```python
from build123d import *

# Parameters (mm, degrees)
BASPROSKE_W        = 10
BASPROSKE_H        = 14
TOOTHCUT_DEPTH     = 23.181073013
TEETHCUTS_COUNT    = 26
TEETHCUTS_ANGLE    = 346.153846154
BORSKE_R           = 0.4
BORE_DEPTH         = 50.0000508
SKETCH1_R          = 8.54
CUT_EXTRUDE1_DEPTH = 5.5
SKETCH2_R          = 3.75
CUT_EXTRUDE2_DEPTH = 21.500522978
SKETCH3_R          = 15.294835459
CUT_EXTRUDE3_DEPTH = 2


with BuildPart() as part:
    # BasProSke → Base-Revolve (revolve)
    with BuildSketch(Plane(origin=(0, 0, 0), x_dir=(1, 0, 0), z_dir=(0, 1, 0)), mode=Mode.PRIVATE) as base_revolve_sk:
        with Locations((5, 7)):
            Rectangle(BASPROSKE_W, BASPROSKE_H)
    revolve(base_revolve_sk.sketch.rotate(Axis((-10, 0, 0), (1, 0, 0)), 180), axis=Axis((-10, 0, 0), (1, 0, 0)))

    # TooCutSke → ToothCut (cut, through all)
    with BuildSketch(Plane(origin=(0, 0, 0), x_dir=(0, 0, -1), z_dir=(1, 0, 0))):
        with BuildLine():
            ThreePointArc((0.476965065, 11.739314517), (0, 11.749), (-0.476965065, 11.739314517))
            ThreePointArc((-0.476965065, 11.739314517), (-0.82065865, 12.901686978), (-1.424117301, 13.952911348))
            ThreePointArc((-1.424117301, 13.952911348), (0, 14.0254), (1.424117301, 13.952911348))
            ThreePointArc((1.424117301, 13.952911348), (0.82065865, 12.901686978), (0.476965065, 11.739314517))
        make_face()
    toothcut = extrude(amount=TOOTHCUT_DEPTH, mode=Mode.SUBTRACT)

    # TeethCuts: ToothCut ×26 about axis
    teethcuts_axis = Axis((-10, 0, 0), (1, 0, 0))
    for i in range(1, TEETHCUTS_COUNT):
        add(toothcut.rotate(teethcuts_axis, i * TEETHCUTS_ANGLE / (TEETHCUTS_COUNT - 1)), mode=Mode.SUBTRACT)

    # BorSke → Bore (cut, symmetric)
    with BuildSketch(Plane(origin=(0, 0, 0), x_dir=(0, 0, -1), z_dir=(1, 0, 0))):
        with Locations(Location((0, 0, 0), (0, 0, 180))):
            Circle(BORSKE_R)
    extrude(amount=BORE_DEPTH, both=True, mode=Mode.SUBTRACT)

    # Sketch1 → Cut-Extrude1 (cut)
    with BuildSketch(Plane(origin=(10, 0, 0), x_dir=(0, 0, -1), z_dir=(1, 0, 0))):
        Circle(SKETCH1_R)
    extrude(amount=-CUT_EXTRUDE1_DEPTH, mode=Mode.SUBTRACT)

    # Sketch2 → Cut-Extrude2 (cut, through all)
    with BuildSketch(Plane(origin=(4.5, 0, 0), x_dir=(0, 0, -1), z_dir=(1, 0, 0))):
        Circle(SKETCH2_R)
    extrude(amount=-CUT_EXTRUDE2_DEPTH, mode=Mode.SUBTRACT)

    # Sketch3 → Cut-Extrude3 (cut)
    with BuildSketch(Plane.ZY):
        Circle(SKETCH3_R)
    extrude(amount=-CUT_EXTRUDE3_DEPTH, mode=Mode.SUBTRACT)


solid = part.part
```
Here's how the part is built. I have some questions about the finished solid (model axes, mm). A direction names the side the tool comes from. Round coordinates to 2 decimals unless told otherwise and drop trailing zeros. Loops run counter-clockwise (first coordinate to the right, second up) from the corner with the lowest first, then second, coordinate; pieces in that order, holes last. Notation, with made-up numbers: (5.25, 21) -> (50.25, 21) arc R13 cw to (50.25, 41) -> close; hole circle Ø5 at (-34, 81.25). An arc over 180 degrees is marked (long way). Answer as CSV lines item,"result".
1. For pin 1 (4 mm diameter, centred on x = 3.5, y = -9.5, fed in from -Z); pin 2 (8.5 mm diameter, centred on y = 0.5, z = 2.5, fed in from +X); pin 3 (3 mm diameter, centred on x = 8.5, z = 6, fed in from -Y), each with a flat end and sliding along its axis, tell me the tip position at first contact or that it passes through.
Final values:
pin 1,"stops at z = -10.66"
pin 2,"stops at x = 4.5"
pin 3,"stops at y = -13.19"
2. If we section it at B-B on y = -8: Please give me the cut outline in (x, z), plus the area to 3 significant figures.
Final values:
outline,"(2, -10.15) -> (10, -10.15) -> (10, -2.99) -> (4.5, -2.99) -> (4.5, 2.99) -> (10, 2.99) -> (10, 10.15) -> (2, 10.15) -> close"
area,"130 mm^2"
3. Thinking about a two-plate mould opening in Y: for faces 5 (the face through (5.944, -12.873, -0.808)), 6 (the face through (5.944, 11.774, -5.266)), which applies, released by +Y, released by -Y, zero draft, split by the parting line, or undercut?
Final values:
face 5,"released by -Y"
face 6,"undercut"
4. If we section it at A-A on z = 0: Please give me the cut outline in (x, y), plus the area to 3 significant figures.
Final values:
outline,"(2, -11.75) -> (10, -11.75) -> (10, -8.54) -> (4.5, -8.54) -> (4.5, -3.75) -> (2, -3.75) -> close; (2, 3.75) -> (4.5, 3.75) -> (4.5, 8.54) -> (10, 8.54) -> (10, 11.75) -> (2, 11.75) -> close"
area,"75.3 mm^2"
5. If I drill on L1, parallel to Y at x = 6.85, z = 0; L2, parallel to Y at x = 2.7, z = 0; L3, parallel to Y at x = 8.25, z = -12, over which ranges is the centre line in solid material (lowest first)?
Final values:
L1,"y = -11.75 to -8.54, 8.54 to 11.75"
L2,"y = -11.75 to -3.75, 3.75 to 11.75"
L3,"y = -6.76 to -5.58, -3.81 to -2.03, -0.92 to 0.92, 2.03 to 3.81, 5.58 to 6.76"
6. Which directions (+Z, -Z, +X, -X, +Y, -Y) give clear straight access to the entire face, cutting with the end or side of a thin tool? Please do faces 1 (the face through (7.288, 8.467, 1.112)), 2 (the face through (5.94, -3.81, -12.32)), 3 (the face through (5.94, -12.9, 0.82)), 4 (the face through (5.94, -0.75, -12.88)).
Final values:
face 1,"+X"
face 2,"+X, -X"
face 3,"+X, -X, -Y"
face 4,"-Z, +X, -X"
